Here's how the part is built. I have some questions about the finished solid (model axes, mm). A direction names the side the tool comes from. Round coordinates to 2 decimals unless told otherwise and drop trailing zeros. Loops run counter-clockwise (first coordinate to the right, second up) from the corner with the lowest first, then second, coordinate; pieces in that order, holes last. Notation, with made-up numbers: (53.5, -36) -> (73.5, -36) arc R6 ccw to (73.5, -32) -> close; hole circle Ø5 at (87, 87). An arc over 180 degrees is marked (long way). Use one line per item in the form item = value. Start each with the question number.
Item 1: If we section it at D-D (y = -4.5): State how many separate pieces and enclosed holes the cut face has, then the cut area to 3 significant figures.
Item 2: If we section it at A-A (z = 1.6): Write out the boundary of the cut face in (x, y), then the cut area to 3 significant figures.
Item 3: For faces 1 (the face through (49.459, 3.275, 1.493)), 2 (the face through (52.564, -20, 1)), which set-ups out of +Z, -Z, +X, -X, +Y, -Y let a thin tool reach every point of the face, with its end or its side?
Item 4: If we section it at B-B (y = -25.5): Write out the boundary of the cut face in (x, z), then the cut area to 3 significant figures.
Item 5: I'm going to push flat-ended pins straight in: pin 1 Ø5.5 at (x, y) = (44.41, -2.23) entering from +Z; pin 2 Ø9.5 at (x, y) = (-6.29, -39.23) entering from +Z. Where does each tip first touch, or does it pass through?
Item 6: If I drill on L1, parallel to X at y = -3, z = 0.75; L2, parallel to Y at x = 33.5, z = 1.15; L3, parallel to X at y = -28, z = 1.3, over which ranges is the centre line in solid material (lowest first)? Write a range as [from, to].
Item 7: If we section it at C-C (x = 25): Write out the boundary of the cut face in (y, z), then the cut area to 3 significant figures.
Item 8: Thinking about a two-plate mould opening in Y: for faces 3 (the face through (49.57, -44.62, 1.49)), 4 (the face through (19, -20, 0)), 5 (the face through (-12.44, -45.624, 1.014)), 6 (the face through (19, -20, 1)), which applies, released by +Y, released by -Y, zero draft, split by the parting line, or undercut?
Autodesk Inventor part; units mm, degrees
ref_plane "YZ Plane" through (0, 0, 0) normal (1, 0, 0) x (0, 1, 0)
ref_plane "XZ Plane" through (0, 0, 0) normal (0, 1, 0) x (-1, 0, 0)
ref_plane "XY Plane" through (0, 0, 0) normal (0, 0, 1) x (1, 0, 0)
sketch "Esboço1" plane through (0, 0, 0) normal (0, 0, 1) x (1, 0, 0)
  line L0 (-14.4362, 6.271) -> (52.5638, 6.271)
  line L1 (52.5638, 6.271) -> (52.5638, -47.729)
  line L2 (52.5638, -47.729) -> (-14.4362, -47.729)
  line L3 (-14.4362, -47.729) -> (-14.4362, 6.271)
  circle A0 centre (-6.2862, -2.229) radius 3
  circle A1 centre (-6.2862, -39.229) radius 3
  circle A2 centre (44.4138, -39.229) radius 3
  circle A3 centre (44.4138, -2.229) radius 3
  point P0 (0, 0)
  dimension "d0" = 67
  dimension "d1" = 54
  dimension "d6" = 6
  dimension "d7" = 6
  dimension "d8" = 6
  dimension "d9" = 6
  dimension "d17" = 50.7
  dimension "d18" = 50.7
  dimension "d19" = 37
  dimension "d20" = 37
  dimension "d21" = 8.15
  dimension "d22" = 8.5
  dimension "d24" = 8.15
  dimension "d26" = 8.5
  dimension "d27" = 8.15
  dimension "d28" = 8.15
  dimension "d29" = 8.5
  dimension "d30" = 8.5
extrude "Extrusão1" add sketch "Esboço1" along normal blind 2
shell "Casca1" thickness 1 removed faces 5 at (11.3623, -15.2254, 2) at (-3.2959, -39.4704, 1.3333) at (-3.2959, -2.4704, 1.3333) at (47.4041, -2.4704, 1.3333) at (47.4041, -39.4704, 1.3333)
chamfer "Chanfro1" distance 1 angle 45 4 edges at (-9.2862, -39.229, 1) (-9.2862, -2.229, 1) (41.4138, -2.229, 1) (41.4138, -39.229, 1)
fillet "Arredondamento1" radius 7 8 edges at (-13.4362, 5.271, 1.5) (-14.4362, 6.271, 1) (52.5638, 6.271, 1) (51.5638, 5.271, 1.5) (51.5638, -46.729, 1.5) (52.5638, -47.729, 1) (-13.4362, -46.729, 1.5) (-14.4362, -47.729, 1)
properties part number "capa de alguma parte da guitarra 2"
Values found:
q1.separate_pieces = 3
q1.enclosed_holes = 0
q1.area = 58.4 mm2
q2.outline = (-14.44, -40.73) arc R7 ccw to (-7.44, -47.73) -> (45.56, -47.73) arc R7 ccw to (52.56, -40.73) -> (52.56, -0.73) arc R7 ccw to (45.56, 6.27) -> (-7.44, 6.27) arc R7 ccw to (-14.44, -0.73) -> close; hole (-13.44, -39.73) arc R7 ccw to (-6.44, -46.73) -> (44.56, -46.73) arc R7 ccw to (51.56, -39.73) -> (51.56, -1.73) arc R7 ccw to (44.56, 5.27) -> (-6.44, 5.27) arc R7 ccw to (-13.44, -1.73) -> close
q2.area = 238 mm2
q3.face_1 = +Z
q3.face_2 = +Z, -Z, +X, +Y, -Y
q4.outline = (-14.44, 0) -> (52.56, 0) -> (52.56, 2) -> (51.56, 2) -> (51.56, 1) -> (-13.44, 1) -> (-13.44, 2) -> (-14.44, 2) -> close
q4.area = 69.0 mm2
q5.pin_1 = through
q5.pin_2 = 1
q6.L1 = [-14.44, -9.96], [-2.62, 40.74], [48.08, 52.56]
q6.L2 = [-47.73, -46.73], [5.27, 6.27]
q6.L3 = [-14.44, -13.44], [51.56, 52.56]
q7.outline = (-47.73, 0) -> (6.27, 0) -> (6.27, 2) -> (5.27, 2) -> (5.27, 1) -> (-46.73, 1) -> (-46.73, 2) -> (-47.73, 2) -> close
q7.area = 56.0 mm2
q8.face_3 = undercut
q8.face_4 = zero draft
q8.face_5 = released by -Y
q8.face_6 = undercut
